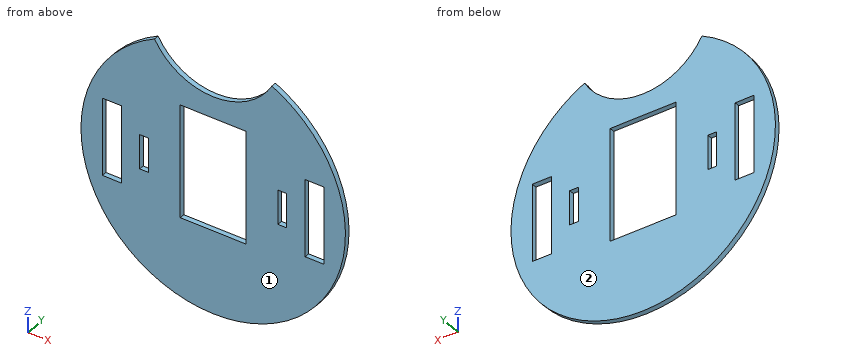
from build123d import *

# Parameters (mm, degrees)
BOSS_EXTRUDE1_DEPTH  = 2.9
SOLENOID_PLACEMENT_W = 37.4
SOLENOID_PLACEMENT_H = 63.8
CUT_EXTRUDE1_DEPTH   = 107.105654892
SKETCH2_W            = 10.76
SKETCH2_H            = 43.707605188
CUT_EXTRUDE2_DEPTH   = 107.105654892
SKETCH3_W            = 5
SKETCH3_H            = 19.4
CUT_EXTRUDE3_DEPTH   = 107.105654892


with BuildPart() as part:
    # Sketch1 → Boss-Extrude1 (new body)
    with BuildSketch(Plane(origin=(0, 0, 0), x_dir=(1, 0, 0), z_dir=(0, 1, 0))):
        with BuildLine():
            ThreePointArc((33.29110537, -67.206415641), (0, 75), (-33.29110537, -67.206415641))
            ThreePointArc((-33.29110537, -67.206415641), (0, -47.791616815), (33.29110537, -67.206415641))
        make_face()
    extrude(amount=BOSS_EXTRUDE1_DEPTH)

    # solenoid placement → Cut-Extrude1 (cut, through all)
    with BuildSketch(Plane(origin=(0, 2.9, 0), x_dir=(1, 0, 0), z_dir=(0, 1, 0))):
        with Locations((0, -3.8)):
            Rectangle(SOLENOID_PLACEMENT_W, SOLENOID_PLACEMENT_H)
    extrude(amount=-CUT_EXTRUDE1_DEPTH, mode=Mode.SUBTRACT)

    # Sketch2 → Cut-Extrude2 (cut, through all)
    with BuildSketch(Plane(origin=(0, 2.9, 0), x_dir=(1, 0, 0), z_dir=(0, 1, 0))):
        with Locations((57.517491988, 0)):
            Rectangle(SKETCH2_W, SKETCH2_H)
        with Locations((-57.517491988, 0)):
            Rectangle(SKETCH2_W, SKETCH2_H)
    extrude(amount=-CUT_EXTRUDE2_DEPTH, mode=Mode.SUBTRACT)

    # Sketch3 → Cut-Extrude3 (cut, through all)
    with BuildSketch(Plane(origin=(0, 2.9, 0), x_dir=(1, 0, 0), z_dir=(0, 1, 0))):
        with Locations((-39.179852803, 0)):
            Rectangle(SKETCH3_W, SKETCH3_H)
        with Locations((39.179852803, 0)):
            Rectangle(SKETCH3_W, SKETCH3_H)
    extrude(amount=-CUT_EXTRUDE3_DEPTH, mode=Mode.SUBTRACT)


solid = part.part
Can you work these out from the model? Positions are in its coordinate system, mm. Face numbers are marked on the shaded views. Round coordinates to 2 decimals unless told otherwise and drop trailing zeros. Write each loop counter-clockwise with the first axis right and the second up, starting at its lowest first coordinate (ties: lowest second). Pieces come first, ordered by that corner, then holes. Notation, with made-up numbers: (63.25, 82.5) -> (112.25, 82.5) arc R19 ccw to (112.25, 119.5) -> close; hole circle Ø8 at (7.5, 51). An arc over 180 degrees is marked (long way). Use one line per item in the form item = value. Start each with the question number.
Q1. If I drill on probe 1 along X at (y, z) = (2.15, -1); probe 2 along X at (y, z) = (0.9, 16.5); probe 3 along X at (y, z) = (1.6, -21.5), over which ranges is the centre line in solid material (lowest first)? Write a range as [from, to].
Q2. Imagine slicing it at B-B (z = 0). Please give me the cut outline in (x, y).
Q3. Imagine slicing it at D-D (z = 25). Please give me the cut outline in (x, y), then the cut area to 3 significant figures.
Q4. Imagine slicing it at A-A (x = 0). Please give me the cut outline in (y, z).
Q5. We'd pull the mould along Y, two halves only. Please class the marked faces 1 and 2: +Y half, -Y half, draft (parallel to the pull), parting line (faces both ways), or undercut.
Q6. I'm going to push flat-ended pins straight in: P1, Ø0.9, axis at x = -58, y = 1, coming from the +Z side; P2, Ø0.9, axis at x = -2, y = 1.5, coming from the -Z side. Where does each tip first touch, or does it pass through?
Q7. Imagine slicing it at C-C (y = 0.65). Please give me the cut outline in (x, z).
Worked out:
q1.probe_1 = [-74.99, -62.9], [-52.14, -41.68], [-36.68, -18.7], [18.7, 36.68], [41.68, 52.14], [62.9, 74.99]
q1.probe_2 = [-73.16, -62.9], [-52.14, -18.7], [18.7, 52.14], [62.9, 73.16]
q1.probe_3 = [-71.85, -62.9], [-52.14, -18.7], [18.7, 52.14], [62.9, 71.85]
q2.outline = (-75, 0) -> (-62.9, 0) -> (-62.9, 2.9) -> (-75, 2.9) -> close; (-52.14, 0) -> (-41.68, 0) -> (-41.68, 2.9) -> (-52.14, 2.9) -> close; (-36.68, 0) -> (-18.7, 0) -> (-18.7, 2.9) -> (-36.68, 2.9) -> close; (18.7, 0) -> (36.68, 0) -> (36.68, 2.9) -> (18.7, 2.9) -> close; (41.68, 0) -> (52.14, 0) -> (52.14, 2.9) -> (41.68, 2.9) -> close; (62.9, 0) -> (75, 0) -> (75, 2.9) -> (62.9, 2.9) -> close
q3.outline = (-70.71, 0) -> (-18.7, 0) -> (-18.7, 2.9) -> (-70.71, 2.9) -> close; (18.7, 0) -> (70.71, 0) -> (70.71, 2.9) -> (18.7, 2.9) -> close
q3.area = 302 mm^2
q4.outline = (0, -75) -> (2.9, -75) -> (2.9, -28.1) -> (0, -28.1) -> close; (0, 35.7) -> (2.9, 35.7) -> (2.9, 47.79) -> (0, 47.79) -> close
q5.face_1 = -Y half
q5.face_2 = +Y half
q6.P1 = 48.09
q6.P2 = -74.98
q7.outline = (-33.29, 67.21) arc R75 ccw (long way) to (33.29, 67.21) arc R38.25 cw to start; hole (-62.9, -21.85) -> (-52.14, -21.85) -> (-52.14, 21.85) -> (-62.9, 21.85) -> close; hole (-41.68, -9.7) -> (-36.68, -9.7) -> (-36.68, 9.7) -> (-41.68, 9.7) -> close; hole (-18.7, -28.1) -> (18.7, -28.1) -> (18.7, 35.7) -> (-18.7, 35.7) -> close; hole (36.68, -9.7) -> (41.68, -9.7) -> (41.68, 9.7) -> (36.68, 9.7) -> close; hole (52.14, -21.85) -> (62.9, -21.85) -> (62.9, 21.85) -> (52.14, 21.85) -> close
